Could you check a few things on this model? Use its own coordinates, in mm. A direction names the side the tool comes from. Give positions to 0.01 mm unless a question says otherwise; leave off trailing zeros. Order: outer loops, then holes, each group sorted by start corner. A loop starts at its lowest first (then second) coordinate and runs counter-clockwise, first axis right, second up.
(1) Imagine slicing it at A-A, the plane z = 1.1. State how many separate pieces and enclosed holes the cut face has, then the cut area to 3 significant figures.
(2) On a 3-axis mill with a long thin cutter (end or side, diameter ignored), from which of +Z, -Z, +X, -X, +Y, -Y can I reach the whole of each face in a straight line? I mean faces 5 (the cylindrical face through (-69.32, 0.5, 2.5)), 6 (the cylindrical face through (-19.065, 26.098, 1.252)). Say none if no direction works.
(3) Will these pins go through, and if not, where does the flat tip stop? pin 1 (2 mm diameter, centred on x = -26, z = 1, fed in from -Y); pin 2 (4.5 mm diameter, centred on x = -34.925, y = 19.05, fed in from +Z); pin 3 (5.5 mm diameter, centred on x = -65.72, y = 4.13, fed in from -Z); pin 4 (1 mm diameter, centred on y = 66.5, z = 4, fed in from -X).
(4) If we mould it in two halves opening along Y, with no side actions, what happens to faces 1 (the flat face through (-36, 45, 0)), 2 (the cylindrical face through (-77.786, 34.448, 2.504)), 3 (the flat face through (-28, 40, 2.54)), 4 (the cylindrical face through (-0.5, 0.53, 2.5))? For each: released by +Y, released by -Y, zero draft, split by the parting line, or undercut.
(5) Imagine slicing it at B-B, the plane y = 19.05. Write out the boundary of the cut face in (x, z), then the cut area to 3 significant figures.
(6) Imagine slicing it at D-D, the plane y = 29. Write out the boundary of the cut face in (x, z), then the cut area to 3 significant figures.
(7) Imagine slicing it at C-C, the plane x = -47.5. Write out the boundary of the cut face in (y, z).
(8) If I drill on probe 1 along X at (y, z) = (14, 2.1); probe 2 along X at (y, z) = (37.5, 0.25); probe 3 along X at (y, z) = (7, 0.45), over which ranges is the centre line in solid material (lowest first)?
Autodesk Inventor part; units mm, degrees
ref_plane "YZ Plane" through (0, 0, 0) normal (1, 0, 0) x (0, 1, 0)
ref_plane "XZ Plane" through (0, 0, 0) normal (0, 1, 0) x (-1, 0, 0)
ref_plane "XY Plane" through (0, 0, 0) normal (0, 0, 1) x (1, 0, 0)
sketch "Sketch1" plane through (0, 0, 0) normal (0, 0, 1) x (1, 0, 0)
  circle A0 centre (-65.7225, 65.7225) radius 3.175
  circle A1 centre (-4.1275, 65.7225) radius 3.175
  circle A2 centre (-4.1275, 4.1275) radius 3.175
  circle A3 centre (-65.7225, 4.1275) radius 3.175
  arc A4 (-67.9183, -0.4854) -> (-1.9317, -0.4854) centre (-34.925, 68.8257) ccw
  arc A5 (-1.9317, 70.3354) -> (-67.9183, 70.3354) centre (-34.925, 1.0243) ccw
  arc A6 (-70.3354, 67.9183) -> (-70.3354, 1.9317) centre (-1.0243, 34.925) ccw
  arc A7 (0.4854, 1.9317) -> (0.4854, 67.9183) centre (-68.8257, 34.925) ccw
  circle A8 centre (-65.7225, 65.7225) radius 5.1089
  circle A9 centre (-4.1275, 65.7225) radius 5.1089
  circle A10 centre (-65.7225, 4.1275) radius 5.1089
  circle A11 centre (-4.1275, 4.1275) radius 5.1089
  arc A12 (-69.85, 62.7118) -> (-69.85, 7.1382) centre (-1.0243, 34.925) ccw
  arc A13 (-7.1382, 69.85) -> (-62.7118, 69.85) centre (-34.925, 1.0243) ccw
  arc A14 (0, 7.1382) -> (0, 62.7118) centre (-68.8257, 34.925) ccw
  arc A15 (-62.7118, 0) -> (-7.1382, 0) centre (-34.925, 68.8257) ccw
  point P0 (0, 0)
  point P1 (-34.925, 77.7875)
  point P2 (-34.925, -7.9375)
  point P3 (-77.7875, 34.925)
  point P4 (7.9375, 34.925)
  point P5 (-34.925, 77.7875)
  point P6 (-34.925, -7.9375)
  dimension "d36" = 6.35
  dimension "d37" = 61.595
  dimension "d38" = 61.595
  dimension "d39" = 85.725
  dimension "d40" = 2.54
  dimension "d41" = 2.54
  dimension "d42" = 2.54
  dimension "d43" = 2.54
  dimension "d44" = 67.8014
  dimension "d45" = 67.8014
extrude "Extrusion1" add sketch "Sketch1" along normal blind 5.08
sketch "Sketch2" plane through (0, 0, 0) normal (0, 0, -1) x (-1, 0, 0)
  circle A0 centre (34.925, 25.4) radius 17.78
  circle A1 centre (34.925, 25.4) radius 15.875
  circle A2 centre (34.925, 19.05) radius 2.0638
  circle A3 centre (34.925, 0) radius 1.5875
  circle A4 centre (34.925, 36.195) radius 4.445
  line L0 (34.925, 40.64) -> (34.925, 31.75)
  circle A5 centre (4.1275, 4.1275) radius 3.175
  circle A6 centre (65.7225, 4.1275) radius 3.175
  circle A7 centre (4.1275, 65.7225) radius 3.175
  circle A8 centre (65.7225, 65.7225) radius 3.175
  arc A9 (1.9317, -0.4854) -> (67.9183, -0.4854) centre (34.925, 68.8257) ccw
  arc A10 (67.9183, -0.4854) -> (70.3354, 1.9317) centre (65.7225, 4.1275) ccw
  arc A11 (70.3354, 1.9317) -> (70.3354, 67.9183) centre (1.0243, 34.925) ccw
  arc A12 (70.3354, 67.9183) -> (67.9183, 70.3354) centre (65.7225, 65.7225) ccw
  arc A13 (67.9183, 70.3354) -> (1.9317, 70.3354) centre (34.925, 1.0243) ccw
  arc A14 (1.9317, 70.3354) -> (-0.4854, 67.9183) centre (4.1275, 65.7225) ccw
  arc A15 (-0.4854, 67.9183) -> (-0.4854, 1.9317) centre (68.8257, 34.925) ccw
  arc A16 (-0.4854, 1.9317) -> (1.9317, -0.4854) centre (4.1275, 4.1275) ccw
  line L1 (50.8794, 25.4) -> (50.8794, 6.1059)
  arc A17 (50.8794, 25.4) -> (18.9706, 25.4) centre (34.925, 25.4) ccw
  line L2 (18.9706, 6.1059) -> (18.9706, 25.4)
  spline S0 degree 3 poles (14.9225, 8.7528) (15.0016, 8.6923) (15.081, 8.6322) (15.1606, 8.5725) (15.5075, 8.3124) (15.8596, 8.059) (16.5735, 7.5663) (16.9354, 7.3271) (17.3017, 7.0951) (17.668, 6.8631) (18.039, 6.6383) (18.5987, 6.3141) (18.7842, 6.2091) (18.9706, 6.1059) knots -0.55013 -0.55013 -0.55013 -0.55013 -0.52027 -0.52027 -0.52027 -0.390203 -0.390203 -0.260135 -0.260135 -0.260135 -0.130068 -0.130068 -0.066158 -0.066158 -0.066158 -0.066158
  line L3 (14.9225, 8.7528) -> (14.9225, 25.4)
  arc A18 (54.9275, 25.4) -> (14.9225, 25.4) centre (34.925, 25.4) ccw
  line L4 (54.9275, 25.4) -> (54.9275, 8.7528)
  spline S1 degree 3 poles (50.8794, 6.1059) (51.0658, 6.2091) (51.2512, 6.3141) (51.811, 6.6383) (52.182, 6.8631) (52.5483, 7.0951) (52.9146, 7.3271) (53.2764, 7.5663) (53.9904, 8.059) (54.3425, 8.3124) (54.6894, 8.5725) (54.769, 8.6322) (54.8484, 8.6923) (54.9275, 8.7528) knots -0.454112 -0.454112 -0.454112 -0.454112 -0.390203 -0.390203 -0.260135 -0.260135 -0.260135 -0.130068 -0.130068 0 0 0 0.029861 0.029861 0.029861 0.029861
  point P0 (34.925, 36.195)
  dimension "d10" = 1.905
  dimension "d11" = 35.56
  dimension "d15" = 4.1275
  dimension "d18" = 3.175
  dimension "d19" = 19.05
  dimension "d21" = 17.145
  dimension "d22" = 8.89
  dimension "d46" = 10.795
  dimension "d47" = 6.35
extrude "Extrusion2" cut sketch "Sketch2" against normal blind 2.54 contours A0 L1 A17 L2 | L2 A17 L1 A0
extrude "Extrusion3" cut sketch "Sketch2" along normal through all both and the other way through all contours A2 | A3
revolve "Revolution1" cut sketch "Sketch2" angle 360 about axis through (-34.925, 40.64, 0) along (0, -1, 0) picked at (34.5704, 34.7564) contours L0 A4
properties part number "Between Seal 1764"
Answer block:
1. separate pieces: 2
1. enclosed holes: 8
1. area: 5,920 mm2
2. face 5: +Z, -Z, -X, -Y
2. face 6: -Z
3. pin 1: stops at y = -7.53
3. pin 2: stops at z = 5.08
3. pin 3: passes through
3. pin 4: stops at x = -71.22
4. face 1: zero draft
4. face 2: split by the parting line
4. face 3: undercut
4. face 4: released by -Y
5. outline: (-76.13, 0) - (-51.53, 0) - (-51.53, 2.54) - (-49.47, 2.54) - (-49.47, 0) - (-36.99, 0) - (-36.99, 5.08) - (-76.13, 5.08) - close; (-32.86, 0) - (-20.38, 0) - (-20.38, 2.54) - (-18.32, 2.54) - (-18.32, 0) - (6.28, 0) - (6.28, 5.08) - (-32.86, 5.08) - close
5. area: 387 mm2
6. outline: (-77.56, 0) - (-52.34, 0) - (-52.34, 2.54) - (-50.39, 2.54) - (-50.39, 0) - (-19.46, 0) - (-19.46, 2.54) - (-17.51, 2.54) - (-17.51, 0) - (7.71, 0) - (7.71, 5.08) - (-77.56, 5.08) - close
6. area: 423 mm2
7. outline: (-6.9, 0) - (12.83, 0) - (12.83, 2.54) - (15.71, 2.54) - (15.71, 0) - (35.09, 0) - (35.09, 2.54) - (37.97, 2.54) - (37.97, 0) - (76.75, 0) - (76.75, 5.08) - (-6.9, 5.08) - close
8. probe 1: x = -74.88 to -48.57, -45.97 to -23.88, -21.28 to 5.03
8. probe 2: x = -77.74 to -47.95, -45.2 to -39.17, -30.68 to -24.65, -21.9 to 7.89
8. probe 3: x = -72.53 to -67.08, -64.37 to -5.48, -2.77 to 2.68
